```python
from build123d import *

# Parameters (mm, degrees)
F0_W     = 50
F0_H     = 20
F1_DEPTH = 3
F2_R     = 4.5
F3_DEPTH = 3.001
F5_DEPTH = 3


with BuildPart() as f1:
    # F0 (on Front) → F1 (new body)
    with BuildSketch(Plane.XZ):
        with Locations((25, 10)):
            Rectangle(F0_W, F0_H)
    extrude(amount=F1_DEPTH)

    # F2 (on face) → F3 (cut, through all)
    with BuildSketch(Plane.XZ.offset(3)):
        with Locations((10, 10)):
            Circle(F2_R)
        with Locations((33.5, 10)):
            Circle(F2_R)
    extrude(amount=-F3_DEPTH, mode=Mode.SUBTRACT)

    # F4 (on face) → F5 (join, through all)
    with BuildSketch(Plane.XZ.offset(3)):
        Polygon((50, 20), (50, 0), (90.476949, 115.33643), (104.084845, 125.385415), (102.314374, 141.059241), (77.317478, 138.235662), (35.823053, 20), align=None)
    extrude(amount=-F5_DEPTH)


solid = f1.part
```
Model file for the job. Use its own axes, mm. A direction names the side the tool comes from. Coordinates: 2 decimals unless noted, no trailing zeros. Loops run counter-clockwise (first coordinate to the right, second up) from the corner with the lowest first, then second, coordinate; pieces in that order, holes last. Notation, with made-up numbers: (48.25, 7.25) - (89.25, 7.25) arc R22 cw to (89.25, 24.25) - close; hole circle Ø2 at (56, -26). An arc over 180 degrees is marked (long way). Answer as a JSON object with one key per item and string values. Group by question number.
(1) Cut at A-A (x = 10). Give the cut face in (y, z), then the cut area to 3 significant figures.
(2) Cut at B-B (z = 10). Give the cut face in (x, y), then the cut area to 3 significant figures.
(3) Flat gauge pins, fed straight in: pin 1 (10.5 mm diameter, centred on x = 10, z = 10, fed in from +Y); pin 2 (1.5 mm diameter, centred on y = -2.5, z = 38.5, fed in from -X); pin 3 (1.5 mm diameter, centred on x = 21.5, y = -2, fed in from +Z). Where does each tip first touch, or does it go through?
(4) Two-plate mould, pull along Z, no slides. Class faces 3 (the face through (37.792, -1.521, 11.352)), 4 (the face through (0, -1, 10)), 5 (the face through (89.991, -1.521, 139.667)): released by +Z, released by -Z, zero draft, split by the parting line, or undercut.
(5) Probe line 1 along Z through (x, y) = (10, -1.15); line 2 along Z through (x, y) = (31, -0.6); line 3 along X through (y, z) = (-0.45, 53). List the from-to ranges inside material, lowest first.
(6) Tool access for faces 1 (the face through (14.292, -1.521, 11.352)), 2 (the face through (18, -1, 20)): list every direction of +Z, -Z, +X, -X, +Y, -Y with a clear straight run to the whole face (end or side of a thin tool).
(7) Cut at D-D (x = 83). Give the cut face in (y, z), then the cut area to 3 significant figures.
(8) Cut at C-C (y = -2.2). Give the cut face in (x, z).
Geometry says:
{
 "1": {"outline": "(-3, 0) - (0, 0) - (0, 5.5) - (-3, 5.5) - close; (-3, 14.5) - (0, 14.5) - (0, 20) - (-3, 20) - close", "area": "33.0 mm^2"},
 "2": {"outline": "(0, -3) - (5.5, -3) - (5.5, 0) - (0, 0) - close; (14.5, -3) - (29, -3) - (29, 0) - (14.5, 0) - close; (38, -3) - (53.51, -3) - (53.51, 0) - (38, 0) - close", "area": "107 mm^2"},
 "3": {"pin 1": "stops at y = 0", "pin 2": "stops at x = 42.05", "pin 3": "stops at z = 20"},
 "4": {"face 3": "undercut", "face 4": "zero draft", "face 5": "released by +Z"},
 "5": {"line 1": "z = 0 to 5.5, 14.5 to 20", "line 2": "z = 0 to 6.26, 13.74 to 20", "line 3": "x = 47.4 to 68.6"},
 "6": {"face 1": "+Y, -Y", "face 2": "+Z, -X, +Y, -Y"},
 "7": {"outline": "(-3, 94.03) - (0, 94.03) - (0, 138.88) - (-3, 138.88) - close", "area": "135 mm^2"},
 "8": {"outline": "(0, 0) - (50, 0) - (90.48, 115.34) - (104.08, 125.39) - (102.31, 141.06) - (77.32, 138.24) - (35.82, 20) - (0, 20) - close; hole circle Ø9 at (10, 10); hole circle Ø9 at (33.5, 10)"}
}
